CAD build for the part. Positions are in the model's coordinates, mm. Face numbers are marked on the shaded views. A direction names the side the tool comes from. Give positions to 0.01 mm unless a question says otherwise; leave off trailing zeros. Loops run counter-clockwise (first coordinate to the right, second up) from the corner with the lowest first, then second, coordinate; pieces in that order, holes last.
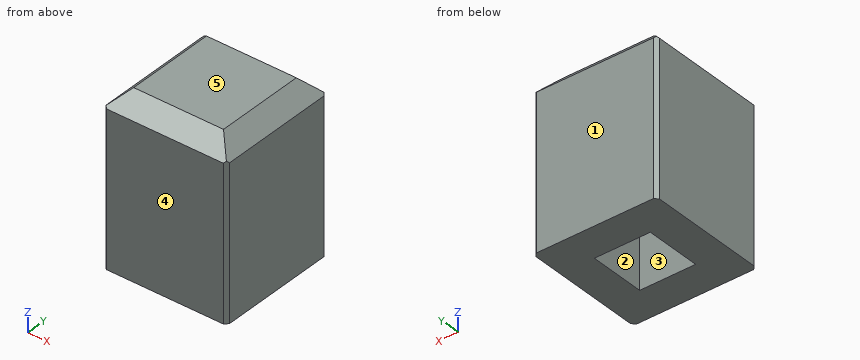
```python
from build123d import *

# Parameters (mm, degrees)
SKETCH1_W           = 7.3
SKETCH1_H           = 7.3
SKETCH1_W_2         = 3.3
SKETCH1_H_2         = 3.3
BOSS_EXTRUDE1_DEPTH = 8
SKETCH3_W           = 7.3
SKETCH3_H           = 7.3
BOSS_EXTRUDE2_DEPTH = 2
CHAMFER1_SIZE       = 1
CHAMFER2_SIZE       = 0.2


with BuildPart() as part:
    # Sketch1 → Boss-Extrude1 (new body)
    with BuildSketch(Plane.XY):
        with Locations((1.65, 1.65)):
            Rectangle(SKETCH1_W, SKETCH1_H)
        with Locations((1.65, 1.65)):
            Rectangle(SKETCH1_W_2, SKETCH1_H_2, mode=Mode.SUBTRACT)
    extrude(amount=BOSS_EXTRUDE1_DEPTH)

    # Sketch3 → Boss-Extrude2 (add)
    with BuildSketch(Plane.XY.offset(8)):
        with Locations((1.65, 1.65)):
            Rectangle(SKETCH3_W, SKETCH3_H)
    extrude(amount=BOSS_EXTRUDE2_DEPTH)

    # Chamfer1
    chamfer1_edges = [part.edges().sort_by_distance(p)[0] for p in [
        (-2, 1.65, 10),
        (1.65, -2, 10),
        (5.3, 1.65, 10),
        (1.65, 5.3, 10),
    ]]
    chamfer(chamfer1_edges, length=CHAMFER1_SIZE)

    # Chamfer2
    chamfer2_edges = [part.edges().sort_by_distance(p)[0] for p in [
        (-2, 5.3, 4.5),
        (5.3, 5.3, 4.5),
        (5.3, -2, 4.5),
        (-2, -2, 4.5),
    ]]
    chamfer(chamfer2_edges, length=CHAMFER2_SIZE)


solid = part.part
```
1. Tool access for the marked faces 1 and 2: list every direction of +Z, -Z, +X, -X, +Y, -Y with a clear straight run to the whole face (end or side of a thin tool).
Responses:
face 1: +Z, -Z, +X, -X, +Y
face 2: -Z
2. Drop a flat-ended pin along its axis: pin 1 (1.6 mm diameter, centred on x = 2, y = 2, fed in from -Z). Give the stop position or say it passes through.
Responses:
pin 1: stops at z = 8
3. Probe line 1 along X through (y, z) = (1, 3.5); line 2 along Z through (x, y) = (1.75, 1.25). List the from-to ranges inside material, lowest first.
Responses:
line 1: x = -2 to 0, 3.3 to 5.3
line 2: z = 8 to 10
4. Saw through at A-A, the plane x = 1.25. List the corners of the cut face in (y, z).
Responses:
outline: (-2, 0) - (0, 0) - (0, 8) - (3.3, 8) - (3.3, 0) - (5.3, 0) - (5.3, 9) - (4.3, 10) - (-1, 10) - (-2, 9) - close
5. Pull direction Y, two halves, no side cores. Call the marked faces 3, 4 and 5: released by +Y, released by -Y, zero draft, split by the parting line, or undercut.
Responses:
face 3: undercut
face 4: released by -Y
face 5: zero draft
6. Saw through at B-B, the plane z = 1. List the corners of the cut face in (x, y), and give its area (3 significant figures).
Responses:
outline: (-2, -1.8) - (-1.8, -2) - (5.1, -2) - (5.3, -1.8) - (5.3, 5.1) - (5.1, 5.3) - (-1.8, 5.3) - (-2, 5.1) - close; hole (0, 0) - (3.3, 0) - (3.3, 3.3) - (0, 3.3) - close
area: 42.3 mm2
